Geometry check sheet. Reference: the model listing, model coordinates, mm. Face numbers are marked on the shaded views. A direction names the side the tool comes from. Coordinates: 2 decimals unless noted, no trailing zeros. Order: outer loops, then holes, each group sorted by start corner. A loop starts at its lowest first (then second) coordinate and runs counter-clockwise, first axis right, second up. Notation, with made-up numbers: (9, -34) - (26, -34) arc R18 ccw to (26, -2) - close; hole circle Ø9 at (8, -7.75). An arc over 180 degrees is marked (long way). Use CSV: the item, a comma, the result in double quotes. Start each with the question number.
1) Draft check along X on the marked faces 3, 4 and 5. Enter one of: released by +X, released by -X, zero draft, split by the parting line, or undercut.
2) Tool access check on the marked faces 1 and 2. Record the directions out of +Z, -Z, +X, -X, +Y, -Y that give a thin tool (end or side, any length) a straight path to the whole face; none if there is none.
3) Sectioned sample at B-B, the plane x = 55. Record the cut outline in (y, z).
4) Sectioned sample at A-A, the plane y = 8.6. Count the separate pieces of the cut face and the enclosed holes in it, and give its area (3 significant figures).
5) Thickness scan on probe 1 along X at (y, z) = (2.4, 6.9); probe 2 along Z at (x, y) = (75, 2.5); probe 3 along X at (y, z) = (25, 42). Record the ranges inside material, lowest first. Write a range as [from, to].
6) Sectioned sample at C-C, the plane z = 41.5. Record the cut outline in (x, y).
7) Sectioned sample at D-D, the plane x = 30. Record the cut outline in (y, z), and give its area (3 significant figures).
8) Depth check by flat-ended pin: P1, Ø0.8, axis at y = 0.5, z = 28, coming from the +X side; P2, Ø1.6, axis at y = 0, z = 29, coming from the -X side; P3, Ø1.8, axis at x = 7, z = 36.5, coming from the +Y side. Enter the tip coordinate at first touch or a pass-through.
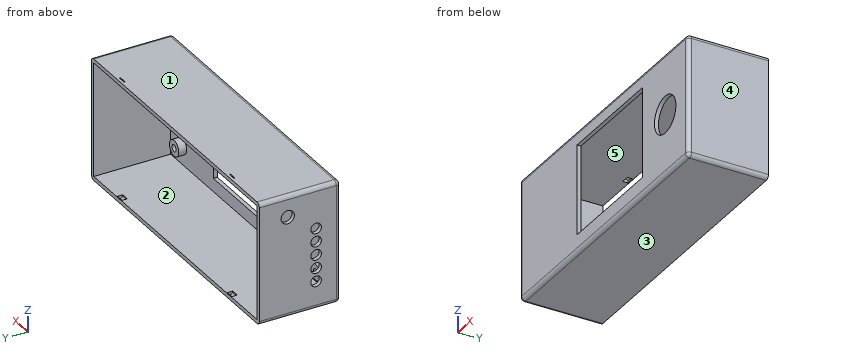
from build123d import *

# Parameters (mm, degrees)
TUBE001_R                  = 3
TUBE001_R_2                = 1.3
TUBE001_DEPTH              = 4
TUBE002_R                  = 3
TUBE002_R_2                = 1.3
TUBE002_DEPTH              = 4
TUBE003_R                  = 3
TUBE003_R_2                = 1.3
TUBE003_DEPTH              = 4
TUBE_R                     = 3
TUBE_R_2                   = 1.3
TUBE_DEPTH                 = 4
CYLINDER007_R              = 2
CYLINDER007_DEPTH          = 10
CYLINDER008_R              = 2
CYLINDER008_DEPTH          = 10
CYLINDER009_R              = 2
CYLINDER009_DEPTH          = 10
CYLINDER010_R              = 2
CYLINDER010_DEPTH          = 10
CYLINDER006_R              = 2
CYLINDER006_DEPTH          = 10
BOX026_W                   = 3
BOX026_H                   = 46
BOX026_DEPTH               = 2
CHAMFER001_SIZE            = 0.9
CHAMFER001_PLACEMENT_ANGLE = 90
BOX025_W                   = 3
BOX025_H                   = 46
BOX025_DEPTH               = 2
CHAMFER_SIZE               = 0.9
CHAMFER_PLACEMENT_ANGLE    = 90
CYLINDER005_R              = 2.5
CYLINDER005_DEPTH          = 10
CYLINDER001_R              = 7
CYLINDER001_DEPTH          = 10
BOX001_W                   = 43
BOX001_H                   = 10
BOX001_DEPTH               = 34
BOX_W                      = 107
BOX_H                      = 29
BOX_DEPTH                  = 43
THICKNESS_T                = 1.5


with BuildPart() as tube001:
    # Tube001 → Tube001 (new body)
    with BuildSketch(Plane(origin=(6.9, 4, 35.9), x_dir=(1, 0, 0), z_dir=(0, -1, 0))):
        Circle(TUBE001_R)
        Circle(TUBE001_R_2, mode=Mode.SUBTRACT)
    extrude(amount=TUBE001_DEPTH)


with BuildPart() as tube002:
    # Tube002 → Tube002 (new body)
    with BuildSketch(Plane(origin=(99.5, 4, 6.9), x_dir=(1, 0, 0), z_dir=(0, -1, 0))):
        Circle(TUBE002_R)
        Circle(TUBE002_R_2, mode=Mode.SUBTRACT)
    extrude(amount=TUBE002_DEPTH)


with BuildPart() as tube003:
    # Tube003 → Tube003 (new body)
    with BuildSketch(Plane(origin=(99.5, 4, 35.9), x_dir=(1, 0, 0), z_dir=(0, -1, 0))):
        Circle(TUBE003_R)
        Circle(TUBE003_R_2, mode=Mode.SUBTRACT)
    extrude(amount=TUBE003_DEPTH)


with BuildPart() as fusion005:
    # Tube → Tube (new body)
    with BuildSketch(Plane(origin=(6.9, 4, 6.9), x_dir=(1, 0, 0), z_dir=(0, -1, 0))):
        Circle(TUBE_R)
        Circle(TUBE_R_2, mode=Mode.SUBTRACT)
    extrude(amount=TUBE_DEPTH)

    # Fusion005: union Tube001, Tube002, Tube003
    add(tube001.part)
    add(tube002.part)
    add(tube003.part)


with BuildPart() as cilindro007:
    # Cylinder007 → Cylinder007 (new body)
    with BuildSketch(Plane(origin=(5.4, 8.6, 24), x_dir=(0, 0, 1), z_dir=(-1, 0, 0))):
        Circle(CYLINDER007_R)
    extrude(amount=CYLINDER007_DEPTH)


with BuildPart() as cilindro008:
    # Cylinder008 → Cylinder008 (new body)
    with BuildSketch(Plane(origin=(5.4, 8.6, 19), x_dir=(0, 0, 1), z_dir=(-1, 0, 0))):
        Circle(CYLINDER008_R)
    extrude(amount=CYLINDER008_DEPTH)


with BuildPart() as cilindro009:
    # Cylinder009 → Cylinder009 (new body)
    with BuildSketch(Plane(origin=(5.4, 8.6, 14), x_dir=(0, 0, 1), z_dir=(-1, 0, 0))):
        Circle(CYLINDER009_R)
    extrude(amount=CYLINDER009_DEPTH)


with BuildPart() as cilindro010:
    # Cylinder010 → Cylinder010 (new body)
    with BuildSketch(Plane(origin=(5.4, 8.6, 9), x_dir=(0, 0, 1), z_dir=(-1, 0, 0))):
        Circle(CYLINDER010_R)
    extrude(amount=CYLINDER010_DEPTH)


with BuildPart() as fusion004:
    # Cylinder006 → Cylinder006 (new body)
    with BuildSketch(Plane(origin=(5.4, 8.6, 29), x_dir=(0, 0, 1), z_dir=(-1, 0, 0))):
        Circle(CYLINDER006_R)
    extrude(amount=CYLINDER006_DEPTH)

    # Fusion004: union Cilindro007, Cilindro008, Cilindro009, Cilindro010
    add(cilindro007.part)
    add(cilindro008.part)
    add(cilindro009.part)
    add(cilindro010.part)


with BuildPart() as chamfer001:
    # Box026 → Box026 (new body)
    with BuildSketch(Plane(origin=(5, -1, -6), x_dir=(1, 0, 0), z_dir=(0, 0, 1))):
        with Locations((1.5, 23)):
            Rectangle(BOX026_W, BOX026_H)
    extrude(amount=BOX026_DEPTH)

    # Chamfer001
    chamfer001_edges = [chamfer001.edges().sort_by_distance(p)[0] for p in [
        (6.5, -1, -6),
        (6.5, -1, -4),
        (6.5, 45, -6),
        (6.5, 45, -4),
    ]]
    chamfer(chamfer001_edges, length=CHAMFER001_SIZE)


with BuildPart() as chamfer001_1:
    # Chamfer001 placement: moved
    add(chamfer001.part.moved(Location((84, 23.7, -0.4))).rotate(Axis((84, 23.7, -0.4), (1, 0, 0)), CHAMFER001_PLACEMENT_ANGLE))


with BuildPart() as fusion:
    # Box025 → Box025 (new body)
    with BuildSketch(Plane(origin=(5, -1, -6), x_dir=(1, 0, 0), z_dir=(0, 0, 1))):
        with Locations((1.5, 23)):
            Rectangle(BOX025_W, BOX025_H)
    extrude(amount=BOX025_DEPTH)

    # Chamfer
    chamfer_edges = [fusion.edges().sort_by_distance(p)[0] for p in [
        (6.5, -1, -6),
        (6.5, -1, -4),
        (6.5, 45, -6),
        (6.5, 45, -4),
    ]]
    chamfer(chamfer_edges, length=CHAMFER_SIZE)


with BuildPart() as fusion_1:
    # Chamfer placement: moved
    add(fusion.part.moved(Location((12, 23.7, -0.4))).rotate(Axis((12, 23.7, -0.4), (1, 0, 0)), CHAMFER_PLACEMENT_ANGLE))

    # Fusion: union Chamfer001
    add(chamfer001_1.part)


with BuildPart() as cilindro005:
    # Cylinder005 → Cylinder005 (new body)
    with BuildSketch(Plane(origin=(3, 19.3, 36.4), x_dir=(0, 0, 1), z_dir=(-1, 0, 0))):
        Circle(CYLINDER005_R)
    extrude(amount=CYLINDER005_DEPTH)


with BuildPart() as cilindro001:
    # Cylinder001 → Cylinder001 (new body)
    with BuildSketch(Plane(origin=(93.75, 1, 21.25), x_dir=(1, 0, 0), z_dir=(0, -1, 0))):
        Circle(CYLINDER001_R)
    extrude(amount=CYLINDER001_DEPTH)


with BuildPart() as cubo001:
    # Box001 → Box001 (new body)
    with BuildSketch(Plane(origin=(36, -1, 5), x_dir=(1, 0, 0), z_dir=(0, 0, 1))):
        with Locations((21.5, 5)):
            Rectangle(BOX001_W, BOX001_H)
    extrude(amount=BOX001_DEPTH)


with BuildPart() as caixa:
    # Box → Box (new body)
    with BuildSketch(Plane.XY):
        with Locations((53.5, 14.5)):
            Rectangle(BOX_W, BOX_H)
    extrude(amount=BOX_DEPTH)

    # Thickness
    thickness_openings = [caixa.faces().sort_by_distance(p)[0] for p in [
        (53.5, 29, 21.5),
    ]]
    offset(amount=THICKNESS_T, openings=thickness_openings)


with BuildPart() as caixa_1:
    # Thickness placement: moved
    add(caixa.part.moved(Location((0, 1, 0))))

    # Cut: cut Cubo001
    add(cubo001.part, mode=Mode.SUBTRACT)

    # Cut001: cut Cilindro001
    add(cilindro001.part, mode=Mode.SUBTRACT)

    # Cut002: cut Cilindro005
    add(cilindro005.part, mode=Mode.SUBTRACT)

    # Cut003: cut Fusion
    add(fusion_1.part, mode=Mode.SUBTRACT)

    # Cut005: cut Fusion004
    add(fusion004.part, mode=Mode.SUBTRACT)

    # Fusion006: union Fusion005
    add(fusion005.part)


solid = caixa_1.part
Evaluation:
1,face 3,"zero draft"
1,face 4,"released by +X"
1,face 5,"undercut"
2,face 1,"+Z, +X, -X, +Y, -Y"
2,face 2,"+Y"
3,outline,"(-0.5, 0) arc R1.5 ccw to (1, -1.5) - (30, -1.5) - (30, 0) - (1, 0) - (1, 5) - (-0.5, 5) - close; (-0.5, 39) - (1, 39) - (1, 43) - (30, 43) - (30, 44.5) - (1, 44.5) arc R1.5 ccw to (-0.5, 43) - close"
4,separate pieces,"5"
4,enclosed holes,"0"
4,area,"427 mm²"
5,probe 1,"[-1.5, 0], [3.9, 5.6], [8.2, 9.9], [96.5, 98.2], [100.8, 102.5], [107, 108.5]"
5,probe 2,"[-1.5, 0], [43, 44.5]"
5,probe 3,"[-1.5, 0], [107, 108.5]"
6,outline,"(-1.5, 1) arc R1.5 ccw to (0, -0.5) - (107, -0.5) arc R1.5 ccw to (108.5, 1) - (108.5, 30) - (107, 30) - (107, 1) - (0, 1) - (0, 30) - (-1.5, 30) - close"
7,outline,"(-0.5, 0) arc R1.5 ccw to (1, -1.5) - (30, -1.5) - (30, 0) - (1, 0) - (1, 43) - (30, 43) - (30, 44.5) - (1, 44.5) arc R1.5 ccw to (-0.5, 43) - close"
7,area,"155 mm²"
8,P1,"x = 108.5"
8,P2,"x = -1.49"
8,P3,"y = 4"
